Geometry: see drawing. Coordinates: mm, zero at the bounding-box minimum. Coordinates: 2 decimals unless noted, no trailing zeros. Loops run counter-clockwise (first coordinate to the right, second up) from the corner with the lowest first, then second, coordinate; pieces in that order, holes last. Notation, with made-up numbers: (-18.75, 60) -> (-14.75, 60) arc R12 ccw to (-14.75, 77) -> close; hole circle Ø7 at (86.25, 30). An arc over 180 degrees is marked (long way). Answer as a JSON object with one key per item and string values.
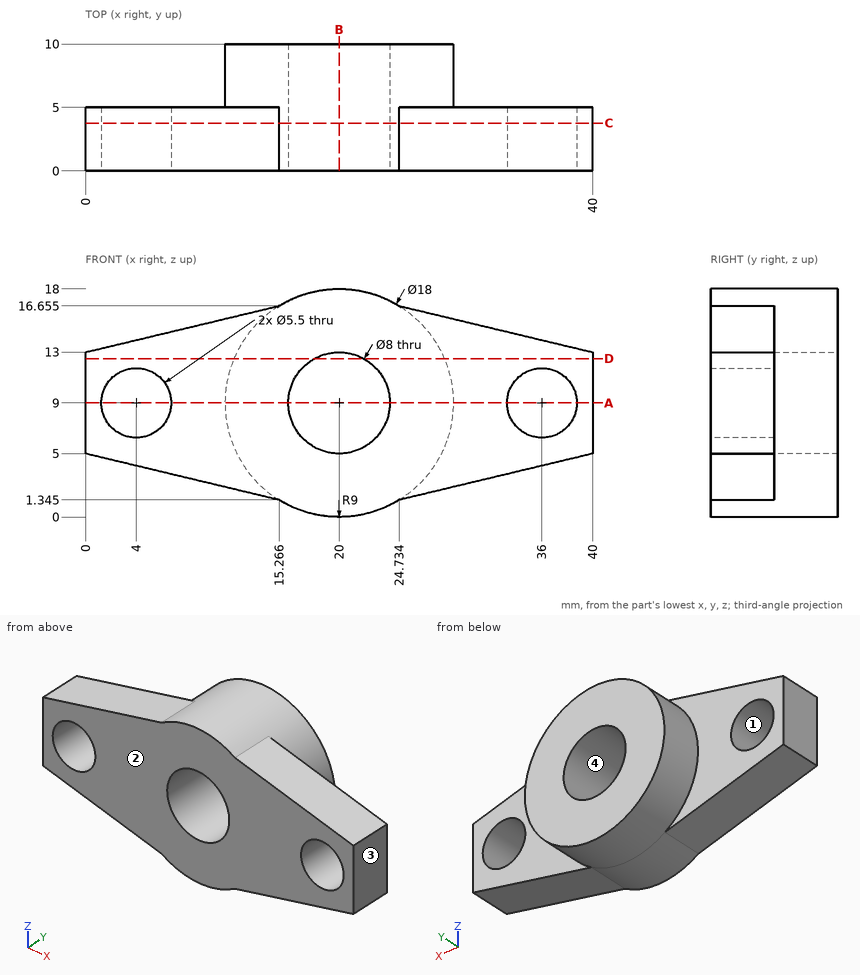
1. Section query A-A (z = 9). Return loops of the section in (x, y), plus the area to 3 significant figures.
Reply:
{"outline": "(0, 0) -> (1.25, 0) -> (1.25, 5) -> (0, 5) -> close; (6.75, 0) -> (16, 0) -> (16, 10) -> (11, 10) -> (11, 5) -> (6.75, 5) -> close; (24, 0) -> (33.25, 0) -> (33.25, 5) -> (29, 5) -> (29, 10) -> (24, 10) -> close; (38.75, 0) -> (40, 0) -> (40, 5) -> (38.75, 5) -> close", "area": "155 mm2"}
2. Section query B-B (x = 20). Return loops of the section in (y, z).
Reply:
{"outline": "(0, 0) -> (10, 0) -> (10, 5) -> (0, 5) -> close; (0, 13) -> (10, 13) -> (10, 18) -> (0, 18) -> close"}
3. Line query: line 1 along X through (y, z) = (1.5, 9); line 2 along X through (y, z) = (0.75, 7.5) (1 decimal); line 3 along X through (y, z) = (8.25, 9). Output: solid intervals per line, ascending.
Reply:
{"line 1": "x = 0 to 1.25, 6.75 to 16, 24 to 33.25, 38.75 to 40", "line 2": "x = 0 to 1.7, 6.3 to 16.3, 23.7 to 33.7, 38.3 to 40", "line 3": "x = 11 to 16, 24 to 29"}
4. Section query C-C (y = 3.75). Count the separate pieces of the cut face and the enclosed holes in it, plus the area to 3 significant figures.
Reply:
{"separate pieces": "1", "enclosed holes": "3", "area": "420 mm2"}
5. Pin query (flat end, axial travel): P1, Ø5, axis at x = 4.5, z = 15.5, coming from the +Y side; P2, Ø1, axis at y = 9, z = 6.5, coming from the +X side (1 decimal); P3, Ø3, axis at x = 34.5, y = 3.5, coming from the +Z side (1 decimal). Return the tip coordinate at first contact, or that it passes through.
Reply:
{"P1": "stops at y = 5", "P2": "stops at x = 28.8", "P3": "stops at z = 14.7"}
6. Mould query, pull axis X, two halves, no side actions, for the marked faces 1, 2, 3 and 4. Classes: pulls with the +X half, pulls with the -X half, needs draft (parallel to the pull), parting line crosses it, or undercut.
Reply:
{"face 1": "undercut", "face 2": "needs draft", "face 3": "pulls with the +X half", "face 4": "undercut"}
7. Section query D-D (z = 12.5). Return loops of the section in (x, y).
Reply:
{"outline": "(0, 0) -> (18.06, 0) -> (18.06, 10) -> (11.71, 10) -> (11.71, 5) -> (0, 5) -> close; (21.94, 0) -> (40, 0) -> (40, 5) -> (28.29, 5) -> (28.29, 10) -> (21.94, 10) -> close"}
